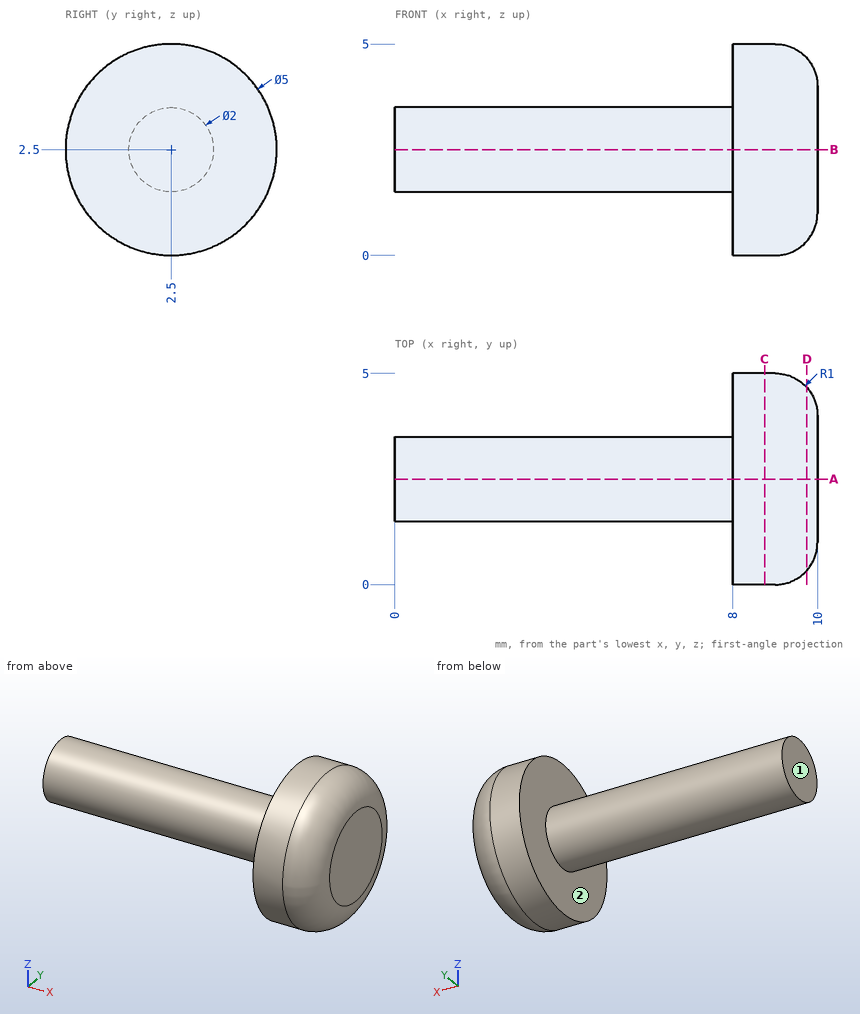
Design review of the part shown in the three views and the two pictorial views. Dimensions are in mm from the part's minimum x, y and z. A direction names the side the tool comes from. Give positions to 0.01 mm unless a question says otherwise; leave off trailing zeros. Write each loop counter-clockwise with the first axis right and the second up, starting at its lowest first coordinate (ties: lowest second). Pieces come first, ordered by that corner, then holes.
(1) Tool access review of the marked faces 1 and 2: name each direction out of +Z, -Z, +X, -X, +Y, -Y from which nothing blocks a thin tool from reaching the whole face with its end or side.
Checked values:
face 1: +Z, -Z, -X, +Y, -Y
face 2: -X
(2) Add section C-C (x = 8.75). Give the boundary of the cut face in (y, z).
Checked values:
outline: circle Ø5 at (2.5, 2.5)
(3) Add section A-A (y = 2.5). Give the boundary of the cut face in (x, z), and give its area (3 significant figures).
Checked values:
outline: (0, 1.5) - (8, 1.5) - (8, 0) - (9, 0) arc R1 ccw to (10, 1) - (10, 4) arc R1 ccw to (9, 5) - (8, 5) - (8, 3.5) - (0, 3.5) - close
area: 25.6 mm2
(4) Wall thickness on line 1 along X through (y, z) = (3, 3.5); line 2 along Z through (x, y) = (9.5, 3.55); line 3 along X through (y, z) = (3.4, 4.5): over which ranges is each line inside the solid? List them lowest first.
Checked values:
line 1: x = 8 to 10
line 2: z = 0.38 to 4.62
line 3: x = 8 to 9.72
(5) Add section D-D (x = 9.75). Give the boundary of the cut face in (y, z), and give its area (3 significant figures).
Checked values:
outline: circle Ø4.32 at (2.5, 2.5)
area: 14.7 mm2
(6) Clearance check with flat-ended pins moving along their axes: pin 1 Ø1 at (x, z) = (5, 3) entering from +Y; pin 2 Ø2 at (x, y) = (1.5, 3) entering from +Z. State where each tip first meets the part, or that it passes through.
Checked values:
pin 1: stops at y = 3.5
pin 2: stops at z = 3.5
